Check sheet for the modelled part. Datum: model origin and axes. Units: mm. Coordinates: 2 decimals unless noted, no trailing zeros. Write each loop counter-clockwise with the first axis right and the second up, starting at its lowest first coordinate (ties: lowest second). Pieces come first, ordered by that corner, then holes. Notation, with made-up numbers: (45, 60.5) -> (99, 60.5) arc R35 ccw to (99, 98.5) -> close; hole circle Ø11 at (-20, 65.5). An arc over 180 degrees is marked (long way). One line per item, written item: value. Start each with the question number.
1) Scan lines: line 1 along X through (y, z) = (5.25, -170.5); line 2 along X through (y, z) = (-1, 137.5); line 3 along Z through (x, y) = (-233.5, -16.25). Record each from-to range of solid material in increasing order. Write a range as [from, to].
2) Sectioned sample at A-A on x = -183. Enter the section's corners in (y, z), plus the area to 3 significant figures.
3) Gauge pin test, flat ends, axial feed: P1, Ø5, axis at x = -15.5, z = -194, coming from the +Y side; P2, Ø5, axis at x = -14.5, y = 5.5, coming from the -Z side; P3, Ø5, axis at x = 232.5, z = 72, coming from the +Y side. Record the tip position at first contact, or that the pin passes through.
4) Sectioned sample at C-C on z = -103. Enter the section's corners in (x, y).
5) Sectioned sample at B-B on y = 5.5. Enter the section's corners in (x, z).
```python
from build123d import *

# Parameters (mm, degrees)
F0_W      = 536
F0_H      = 500
F0_W_2    = 456
F0_H_2    = 450
F1_DEPTH  = 20
F2_W      = 10
F2_H      = 10
F3_DEPTH  = 536
F4_W      = 10
F4_H      = 500
F5_DEPTH  = 10
F6_W      = 10
F6_H      = 10
F7_DEPTH  = 20
F8_W      = 10
F8_H      = 10
F9_DEPTH  = 20
F10_W     = 10
F10_H     = 20
F11_DEPTH = 490
F12_DEPTH = 10
F13_W     = 10
F13_H     = 10
F14_DEPTH = 476


with BuildPart() as f1:
    # F0 (on Front) → F1 (new body)
    with BuildSketch(Plane.XZ):
        with Locations((-8.6522214115, 52.6769706468)):
            Rectangle(F0_W, F0_H)
        with Locations((-8.6522214115, 57.6769706468)):
            Rectangle(F0_W_2, F0_H_2, mode=Mode.SUBTRACT)
    extrude(amount=F1_DEPTH)

    # F2 (on face) → F3 (cut, through all)
    with BuildSketch(Plane(origin=(-276.6522214115, 0, 0), x_dir=(0, -1, 0), z_dir=(-1, 0, 0))):
        with Locations((15, -192.3230293532)):
            Rectangle(F2_W, F2_H)
    extrude(amount=-F3_DEPTH, mode=Mode.SUBTRACT)

    # F4 (on face) → F5 (cut)
    with BuildSketch(Plane(origin=(0, 0, 0), x_dir=(-1, 0, 0), z_dir=(0, 1, 0))):
        with Locations((251.6522214115, 52.6769706468)):
            Rectangle(F4_W, F4_H)
        with Locations((-234.3477785885, 52.6769706468)):
            Rectangle(F4_W, F4_H)
    extrude(amount=-F5_DEPTH, mode=Mode.SUBTRACT)

    # F6 (on face) → F7 (cut, through all)
    with BuildSketch(Plane.YZ.offset(259.3477785885)):
        with Locations((-5, -192.3230293532)):
            Rectangle(F6_W, F6_H)
    extrude(amount=-F7_DEPTH, mode=Mode.SUBTRACT)

    # F8 (on face) → F9 (cut, through all)
    with BuildSketch(Plane(origin=(-276.6522214115, 0, 0), x_dir=(0, -1, 0), z_dir=(-1, 0, 0))):
        with Locations((5, -192.3230293532)):
            Rectangle(F8_W, F8_H)
    extrude(amount=-F9_DEPTH, mode=Mode.SUBTRACT)

    # F10 (on face) → F11 (cut, through all)
    with BuildSketch(Plane.XY.offset(302.6769706468)):
        with Locations((-271.6522214115, -10)):
            Rectangle(F10_W, F10_H)
        with Locations((254.3477785885, -10)):
            Rectangle(F10_W, F10_H)
    extrude(amount=-F11_DEPTH, mode=Mode.SUBTRACT)

    # F12 (add): faces of the model
    f12_faces = [f1.faces().sort_by_distance(p)[0] for p in [
        (222.4443301749, 0, 52.6769706468),
        (244.3477785885, 0, 57.6769706468),
        (-261.6522214115, 0, 57.6769706468),
    ]]
    extrude(f12_faces, amount=F12_DEPTH)

    # F13 (on face) → F14 (cut, through all)
    with BuildSketch(Plane.YZ.offset(229.3477785885)):
        with Locations((5, -192.3230293532)):
            Rectangle(F13_W, F13_H)
    extrude(amount=-F14_DEPTH, mode=Mode.SUBTRACT)


solid = f1.part
```
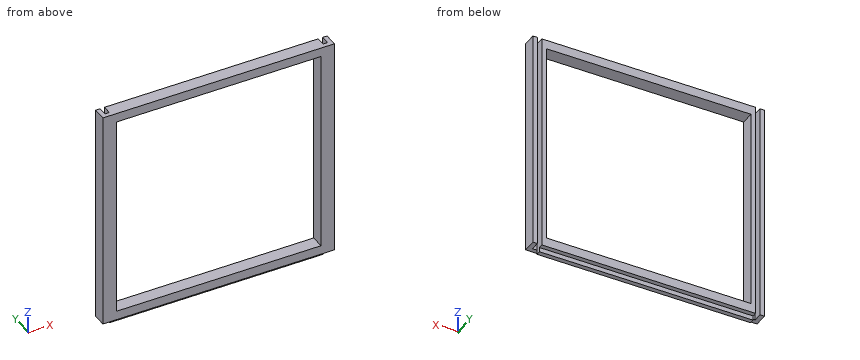
Answers:
1. line 1: x = [-266.65, -256.65], [-246.65, 229.35], [239.35, 249.35]
1. line 2: x = [-266.65, -256.65], [-246.65, -236.65], [219.35, 229.35], [239.35, 249.35]
1. line 3: z = [-187.32, -167.32], [282.68, 302.68]
2. outline: (-20, -187.32) -> (-10, -187.32) -> (-10, -197.32) -> (0, -197.32) -> (0, -187.32) -> (10, -187.32) -> (10, -167.32) -> (-20, -167.32) -> close; (-20, 282.68) -> (10, 282.68) -> (10, 302.68) -> (-20, 302.68) -> close
2. area: 1,300 mm2
3. P1: stops at y = 0
3. P2: stops at z = -187.32
3. P3: stops at y = -10
4. outline: (-266.65, -20) -> (-236.65, -20) -> (-236.65, 10) -> (-246.65, 10) -> (-246.65, -10) -> (-256.65, -10) -> (-256.65, 10) -> (-266.65, 10) -> close; (219.35, -20) -> (249.35, -20) -> (249.35, 10) -> (239.35, 10) -> (239.35, -10) -> (229.35, -10) -> (229.35, 10) -> (219.35, 10) -> close
5. outline: (-266.65, -187.32) -> (-256.65, -187.32) -> (-256.65, 302.68) -> (-266.65, 302.68) -> close; (-246.65, -187.32) -> (229.35, -187.32) -> (229.35, 302.68) -> (-246.65, 302.68) -> close; (239.35, -187.32) -> (249.35, -187.32) -> (249.35, 302.68) -> (239.35, 302.68) -> close; hole (-236.65, -167.32) -> (219.35, -167.32) -> (219.35, 282.68) -> (-236.65, 282.68) -> close
